Read the model definition and answer for the solid it produces. Units are mm, in the model's axes. Face numbers are marked on the shaded views. A direction names the side the tool comes from. Round coordinates to 2 decimals unless told otherwise and drop trailing zeros. Order: outer loops, then holes, each group sorted by start corner. A loop starts at its lowest first (then second) coordinate and runs counter-clockwise, first axis right, second up. Notation, with made-up numbers: (-35.5, 26.5) - (-5.5, 26.5) arc R20 ccw to (-5.5, 37.5) - close; hole circle Ø11 at (-16, 77). An arc over 180 degrees is marked (long way). Put each result on its own line as item: value. Start each with the question number.
Q1. Each of these flat-tipped pins is pushed along its axis until it touches: pin 1 Ø2.5 at (x, z) = (0, 16) entering from +Y; pin 2 Ø6 at (x, z) = (10, 8) entering from -Y; pin 3 Ø5 at (x, y) = (5.5, 1.5) entering from +Z; pin 4 Ø1.7 at (x, z) = (16, 0) entering from +Y. Where does it stop, or does it pass through?
Q2. Which of the six approach directions +Z, -Z, +X, -X, +Y, -Y give full straight-line access (tool end or side, diameter ignored) to the marked faces 1, 2 and 3?
Q3. Section D-D on x = 15.5 is taken. Give the vertices of the cut face in (y, z), then the cut area to 3 significant figures.
Q4. Section B-B on x = 0 is taken. Give the vertices of the cut face in (y, z), then the cut area to 3 significant figures.
Q5. Find the intervals of material crossed by line 1 along Z through (x, y) = (0, -0.4); line 2 along Z through (x, y) = (16, -0.25); line 3 along Z through (x, y) = (8, -0.3), in increasing order. Write a range as from..to.
Q6. Section C-C on z = 15.5 is taken. Give the vertices of the cut face in (x, y).
Q7. Section A-A on z = 0 is taken. Give the vertices of the cut face in (x, y), then the cut area to 3 significant figures.
Autodesk Inventor part; units mm, degrees
ref_plane "YZ Plane" through (0, 0, 0) normal (1, 0, 0) x (0, 1, 0)
ref_plane "XZ Plane" through (0, 0, 0) normal (0, 1, 0) x (-1, 0, 0)
ref_plane "XY Plane" through (0, 0, 0) normal (0, 0, 1) x (1, 0, 0)
sketch "スケッチ1" plane through (0, 0, 0) normal (1, 0, 0) x (0, 1, 0)
  line L0 (0, 0) -> (15, 0)
  line L1 (15, 0) -> (15, -2.75)
  line L2 (15, -2.75) -> (8, -14.25)
  line L3 (8, -14.25) -> (0, -14.25)
  line L4 (0, -14.25) -> (0, 0)
  dimension "d0" = 14.25
  dimension "d1" = 15
  dimension "d2" = 2.75
  dimension "d3" = 8
revolve "回転1" add sketch "スケッチ1" angle 360 about axis through (0, 0, 0) along (0, 1, 0)
sketch "スケッチ2" plane through (0, 0, 0) normal (0, -1, 0) x (1, 0, 0)
  circle A0 centre (0, 16) radius 1.05
  circle A1 centre (0, 8) radius 1.5
  arc A2 (2.0468, 16.1153) -> (-2.0468, 16.1153) centre (0, 16) ccw
  line L0 (2.0468, 16.1153) -> (2.5458, 7.2567)
  line L1 (-2.0468, 16.1153) -> (-2.5458, 7.2567)
  circle A3 centre (0, 0) radius 14.25 construction
  circle A4 centre (0, 8) radius 2.5 construction
  arc A5 (2.5458, 7.2567) -> (7.2567, 2.5458) centre (7.5379, 7.5379) ccw
  circle A6 centre (-16, 0) radius 1.05
  circle A7 centre (-8, 0) radius 1.5
  arc A8 (-16.1153, 2.0468) -> (-16.1153, -2.0468) centre (-16, 0) ccw
  line L2 (-16.1153, 2.0468) -> (-7.2567, 2.5458)
  line L3 (-16.1153, -2.0468) -> (-7.2567, -2.5458)
  circle A9 centre (-8, 0) radius 2.5 construction
  arc A10 (-7.2567, 2.5458) -> (-2.5458, 7.2567) centre (-7.5379, 7.5379) ccw
  circle A11 centre (0, -16) radius 1.05
  circle A12 centre (0, -8) radius 1.5
  arc A13 (-2.0468, -16.1153) -> (2.0468, -16.1153) centre (0, -16) ccw
  line L4 (-2.0468, -16.1153) -> (-2.5458, -7.2567)
  line L5 (2.0468, -16.1153) -> (2.5458, -7.2567)
  circle A14 centre (0, -8) radius 2.5 construction
  arc A15 (-2.5458, -7.2567) -> (-7.2567, -2.5458) centre (-7.5379, -7.5379) ccw
  circle A16 centre (16, 0) radius 1.05
  circle A17 centre (8, 0) radius 1.5
  arc A18 (16.1153, -2.0468) -> (16.1153, 2.0468) centre (16, 0) ccw
  line L6 (16.1153, -2.0468) -> (7.2567, -2.5458)
  line L7 (16.1153, 2.0468) -> (7.2567, 2.5458)
  circle A19 centre (8, 0) radius 2.5 construction
  arc A20 (7.2567, -2.5458) -> (2.5458, -7.2567) centre (7.5379, -7.5379) ccw
  point P0 (7.2567, 2.5458)
  dimension "d5" = 2.1
  dimension "d6" = 3
  dimension "d7" = 16
  dimension "d8" = 1
  dimension "d9" = 1
  dimension "d10" = 5
  dimension "d13" = 360
  dimension "d15" = 8
extrude "押し出し1" add sketch "スケッチ2" along normal blind 0.7
properties part number "MainMotor._Newipt"
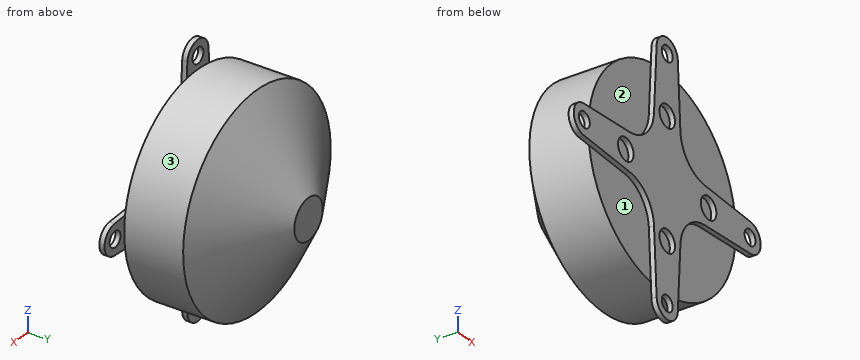
Findings:
1. pin 1: y = 0
1. pin 2: y = 0
1. pin 3: z = 13.93
1. pin 4: through
2. face 1: -Z, -X, -Y
2. face 2: +Z, -X, -Y
2. face 3: +Y
3. outline: (-0.7, -2.08) - (0, -2.08) - (0, -0.92) - (-0.7, -0.92) - close; (-0.7, 0.92) - (0, 0.92) - (0, 2.08) - (-0.7, 2.08) - close
3. area: 1.62 mm2
4. outline: (-0.7, -18.05) - (0, -18.05) - (0, -17.05) - (-0.7, -17.05) - close; (-0.7, -14.95) - (0, -14.95) - (0, -14.25) - (8, -14.25) - (15, -2.75) - (15, 2.75) - (8, 14.25) - (0, 14.25) - (0, 14.95) - (-0.7, 14.95) - (-0.7, 9.5) - (0, 9.5) - (0, 6.5) - (-0.7, 6.5) - (-0.7, -6.5) - (0, -6.5) - (0, -9.5) - (-0.7, -9.5) - close; (-0.7, 17.05) - (0, 17.05) - (0, 18.05) - (-0.7, 18.05) - close
4. area: 365 mm2
5. line 1: -18.05..-17.05, -14.95..-9.5, -6.5..6.5, 9.5..14.95, 17.05..18.05
5. line 2: -2.05..-1.05, 1.05..2.05
5. line 3: -2.5..-1.5, 1.5..2.5
6. outline: (-2.08, -0.7) - (-0.92, -0.7) - (-0.92, 0) - (-2.08, 0) - close; (0.92, -0.7) - (2.08, -0.7) - (2.08, 0) - (0.92, 0) - close
7. outline: (-18.05, -0.7) - (-17.05, -0.7) - (-17.05, 0) - (-18.05, 0) - close; (-14.95, -0.7) - (-9.5, -0.7) - (-9.5, 0) - (-6.5, 0) - (-6.5, -0.7) - (6.5, -0.7) - (6.5, 0) - (9.5, 0) - (9.5, -0.7) - (14.95, -0.7) - (14.95, 0) - (14.25, 0) - (14.25, 8) - (2.75, 15) - (-2.75, 15) - (-14.25, 8) - (-14.25, 0) - (-14.95, 0) - close; (17.05, -0.7) - (18.05, -0.7) - (18.05, 0) - (17.05, 0) - close
7. area: 365 mm2
